Geometry check sheet. Reference: drawing and pictorial views, mm from the part's lowest x, y, z. A direction names the side the tool comes from. Give positions to 0.01 mm unless a question says otherwise; leave off trailing zeros. Loops run counter-clockwise (first coordinate to the right, second up) from the corner with the lowest first, then second, coordinate; pieces in that order, holes last. Notation, with made-up numbers: (67, 10) -> (115, 10) arc R21 cw to (115, 24) -> close; hole circle Ø11 at (33.5, 39.5). An arc over 180 degrees is marked (long way). Answer in a Markdown table with one row per item. Add a question column.
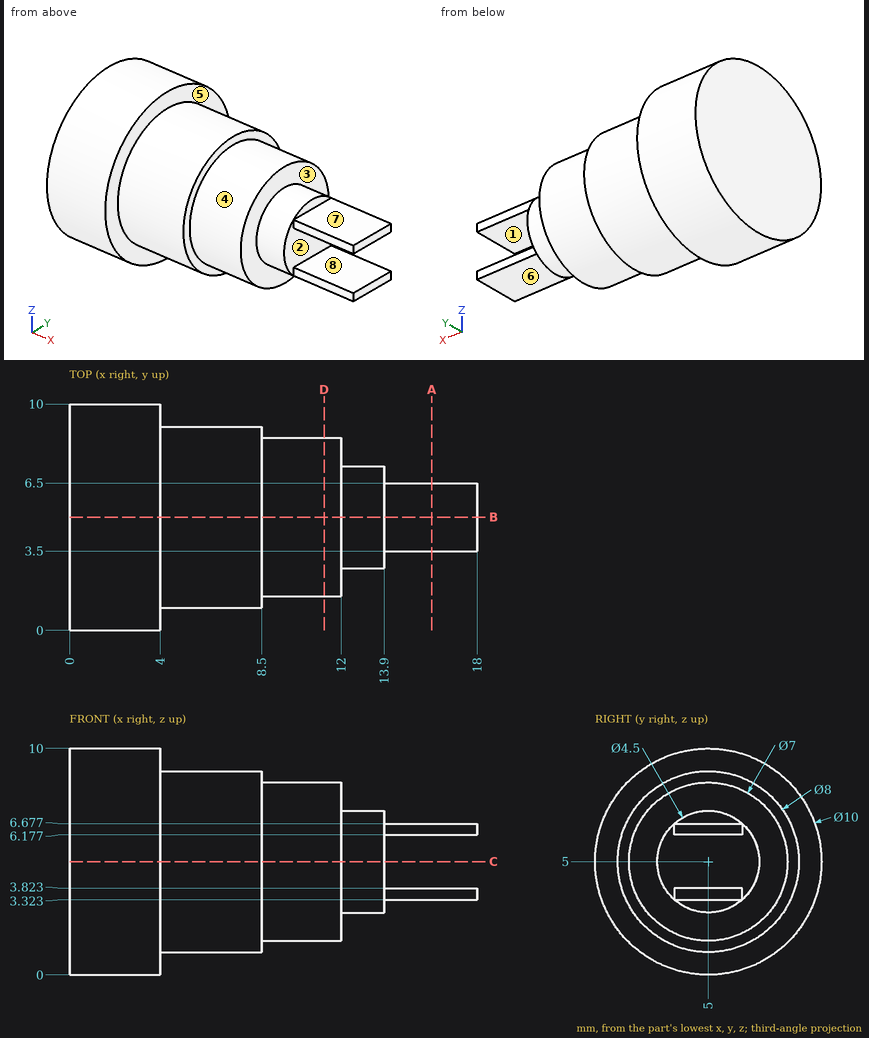
1. Release check for a two-part mould opening along Z. For the marked faces 1, 2, 3 and 4 record: released by +Z, released by -Z, zero draft, split by the parting line, or undercut.
2. Material ranges on L1, parallel to X at y = 3.75, z = 7.25; L2, parallel to X at y = 8, z = 7; L3, parallel to Y at x = 13.25, z = 3.5, recorded low to high. Write a range as from..to.
3. Sectioned sample at B-B (y = 5). Enter the section's corners in (x, z), plus the area to 3 significant figures.
4. Gauge pin test, flat ends, axial feed: pin 1 Ø1 at (y, z) = (4.5, 5.5) entering from +X; pin 2 Ø3.5 at (x, y) = (17, 5.5) entering from -Z; pin 3 Ø0.9 at (x, y) = (16.5, 5.5) entering from +Z. Record the tip position at first contact, or that the pin passes through.
5. Sectioned sample at A-A (x = 16). Enter the section's corners in (y, z).
6. Sectioned sample at D-D (x = 11.25). Enter the section's corners in (y, z).
7. Sectioned sample at C-C (z = 5). Enter the section's corners in (x, y), plus the area to 3 significant figures.
8. Access from +Z, -Z, +X, -X, +Y, -Y to the whole of each face (thin tool, end or side, straight path). Record for the marked faces 5, 6, 7 and 8.
Response:
| question | item | result |
|---|---|---|
| 1 | face 1 | undercut |
| 1 | face 2 | undercut |
| 1 | face 3 | zero draft |
| 1 | face 4 | split by the parting line |
| 2 | L1 | x = 0..12 |
| 2 | L2 | x = 0..8.5 |
| 2 | L3 | y = 3.32..6.68 |
| 3 | outline | (0, 0) -> (4, 0) -> (4, 1) -> (8.5, 1) -> (8.5, 1.5) -> (12, 1.5) -> (12, 2.75) -> (13.9, 2.75) -> (13.9, 3.32) -> (18, 3.32) -> (18, 3.82) -> (13.9, 3.82) -> (13.9, 6.18) -> (18, 6.18) -> (18, 6.68) -> (13.9, 6.68) -> (13.9, 7.25) -> (12, 7.25) -> (12, 8.5) -> (8.5, 8.5) -> (8.5, 9) -> (4, 9) -> (4, 10) -> (0, 10) -> close |
| 3 | area | 113 mm2 |
| 4 | pin 1 | stops at x = 13.9 |
| 4 | pin 2 | stops at z = 3.32 |
| 4 | pin 3 | stops at z = 6.68 |
| 5 | outline | (3.5, 3.32) -> (6.5, 3.32) -> (6.5, 3.82) -> (3.5, 3.82) -> close; (3.5, 6.18) -> (6.5, 6.18) -> (6.5, 6.68) -> (3.5, 6.68) -> close |
| 6 | outline | circle Ø7 at (5, 5) |
| 7 | outline | (0, 0) -> (4, 0) -> (4, 1) -> (8.5, 1) -> (8.5, 1.5) -> (12, 1.5) -> (12, 2.75) -> (13.9, 2.75) -> (13.9, 7.25) -> (12, 7.25) -> (12, 8.5) -> (8.5, 8.5) -> (8.5, 9) -> (4, 9) -> (4, 10) -> (0, 10) -> close |
| 7 | area | 109 mm2 |
| 8 | face 5 | +X |
| 8 | face 6 | -Z, +X, +Y, -Y |
| 8 | face 7 | +Z, +X, +Y, -Y |
| 8 | face 8 | +X, +Y, -Y |
